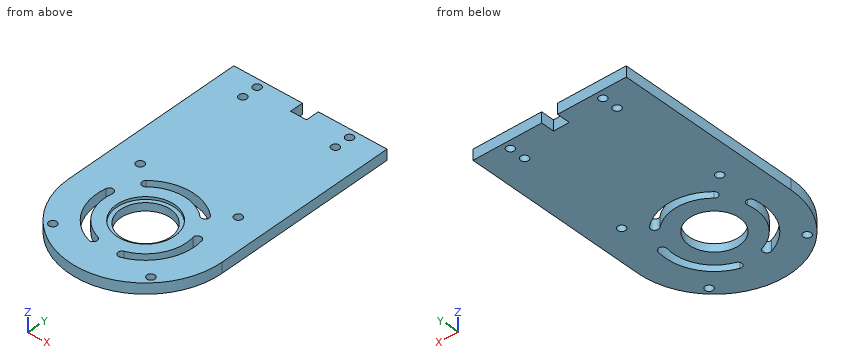
```python
from build123d import *

# Parameters (mm, degrees)
SKETCH_1_R          = 9.525
SKETCH_1_R_2        = 1.5
EXTRUDE_1_DEPTH     = 4
SKETCH_2_W          = 6
SKETCH_2_H          = 5
CUT_EXTRUDE_1_DEPTH = 98.49871794
CUT_EXTRUDE_2_DEPTH = 10
SKETCH_4_R          = 11
CUT_EXTRUDE_3_DEPTH = 1


with BuildPart() as part:
    # 草图1 → 凸台-拉伸1 (new body)
    with BuildSketch(Plane.XY):
        with BuildLine():
            Line((-29, 6), (29, 6))
            Line((29, 6), (29, -64))
            ThreePointArc((29, -64), (0, -93), (-29, -64))
            Line((-29, -64), (-29, 6))
        make_face()
        with Locations((0, -64)):
            Circle(SKETCH_1_R, mode=Mode.SUBTRACT)
        with Locations((-17.5, 3)):
            Circle(SKETCH_1_R_2, mode=Mode.SUBTRACT)
        with Locations((17.5, 3)):
            Circle(SKETCH_1_R_2, mode=Mode.SUBTRACT)
        with Locations((18.561553006, -82.561553006)):
            Circle(SKETCH_1_R_2, mode=Mode.SUBTRACT)
        with Locations((-18.561553006, -82.561553006)):
            Circle(SKETCH_1_R_2, mode=Mode.SUBTRACT)
        with Locations((-18.561553006, -45.438446994)):
            Circle(SKETCH_1_R_2, mode=Mode.SUBTRACT)
        with Locations((18.561553006, -45.438446994)):
            Circle(SKETCH_1_R_2, mode=Mode.SUBTRACT)
        with Locations((-17.5, -3)):
            Circle(SKETCH_1_R_2, mode=Mode.SUBTRACT)
        with Locations((17.5, -3)):
            Circle(SKETCH_1_R_2, mode=Mode.SUBTRACT)
    extrude(amount=EXTRUDE_1_DEPTH)

    # 草图2 → 切除-拉伸1 (cut, through all)
    with BuildSketch(Plane.XY.offset(4)):
        with Locations((0, 3.5)):
            Rectangle(SKETCH_2_W, SKETCH_2_H)
    extrude(amount=-CUT_EXTRUDE_1_DEPTH, mode=Mode.SUBTRACT)

    # 草图3 → 切除-拉伸2 (cut)
    with BuildSketch(Plane.XY.offset(4)):
        with BuildLine():
            ThreePointArc((12.196146044, -50.10328221), (0, -45.510415266), (-12.196146044, -50.10328221))
            ThreePointArc((-12.196146044, -50.10328221), (-12.333149971, -52.20541334), (-10.231018841, -52.342417267))
            ThreePointArc((-10.231018841, -52.342417267), (0, -48.489584734), (10.231018841, -52.342417267))
            ThreePointArc((10.231018841, -52.342417267), (12.333149971, -52.20541334), (12.196146044, -50.10328221))
        make_face()
        with BuildLine():
            ThreePointArc((5.936837613, -81.510531197), (16.012450085, -73.244792367), (18.132983657, -60.386186592))
            ThreePointArc((18.132983657, -60.386186592), (16.38098666, -59.216472147), (15.211272214, -60.968469144))
            ThreePointArc((15.211272214, -60.968469144), (13.432413643, -71.755207633), (4.980253373, -78.68911359))
            ThreePointArc((4.980253373, -78.68911359), (4.047836689, -80.578114513), (5.936837613, -81.510531197))
        make_face()
        with BuildLine():
            ThreePointArc((-18.132983657, -60.386186592), (-16.012450085, -73.244792367), (-5.936837613, -81.510531197))
            ThreePointArc((-5.936837613, -81.510531197), (-4.047836689, -80.578114513), (-4.980253373, -78.68911359))
            ThreePointArc((-4.980253373, -78.68911359), (-13.432413643, -71.755207633), (-15.211272214, -60.968469144))
            ThreePointArc((-15.211272214, -60.968469144), (-16.38098666, -59.216472147), (-18.132983657, -60.386186592))
        make_face()
    extrude(amount=-CUT_EXTRUDE_2_DEPTH, mode=Mode.SUBTRACT)

    # 草图4 → 切除-拉伸3 (cut)
    with BuildSketch(Plane.XY.offset(4)):
        with Locations((0, -64)):
            Circle(SKETCH_4_R)
    extrude(amount=-CUT_EXTRUDE_3_DEPTH, mode=Mode.SUBTRACT)


solid = part.part
```
Input: part model. Units: mm. Frame: model coordinates. Give positions to 0.01 mm unless a question says otherwise; leave off trailing zeros. Order: outer loops, then holes, each group sorted by start corner. A loop starts at its lowest first (then second) coordinate and runs counter-clockwise, first axis right, second up.
1. Cut plane D-D (y = -86). Return loops of the section in (x, z).
Computed:
outline: (-18.89, 0) - (18.89, 0) - (18.89, 4) - (-18.89, 4) - close
2. Cut plane C-C (z = 0.75). State how many separate pieces and enclosed holes the cut face has, and give its area (3 significant figures).
Computed:
separate pieces: 1
enclosed holes: 12
area: 4,770 mm2
3. Cut plane B-B (y = -3). Return loops of the section in (x, z), and give its area (3 significant figures).
Computed:
outline: (-29, 0) - (-19, 0) - (-19, 4) - (-29, 4) - close; (-16, 0) - (16, 0) - (16, 4) - (-16, 4) - close; (19, 0) - (29, 0) - (29, 4) - (19, 4) - close
area: 208 mm2
4. Line query: probe 1 along Y at (x, z) = (6.5, 3.4); probe 2 along X at (y, z) = (-77.5, 0.7); probe 3 along X at (y, z) = (-65, 3.25). Output: solid intervals per line, ascending.
Computed:
probe 1: y = -92.26 to -81.31, -78.08 to -72.87, -55.13 to -49.92, -46.69 to 6
probe 2: x = -25.67 to -12.63, -7.64 to 7.64, 12.63 to 25.67
probe 3: x = -28.98 to -18.46, -15.48 to -10.95, 10.95 to 15.48, 18.46 to 28.98
5. Cut plane A-A (x = 0). Return loops of the section in (y, z) (3 decimals).
Computed:
outline: (-93, 0) - (-73.525, 0) - (-73.525, 3) - (-75, 3) - (-75, 4) - (-93, 4) - close; (-54.475, 0) - (-48.49, 0) - (-48.49, 4) - (-53, 4) - (-53, 3) - (-54.475, 3) - close; (-45.51, 0) - (1, 0) - (1, 4) - (-45.51, 4) - close
6. Pin query (flat end, axial travel): pin 1 Ø20 at (x, y) = (0, -64) entering from +Z. Return the tip coordinate at first contact, or that it passes through.
Computed:
pin 1: stops at z = 3
